Geometry check sheet. Reference: the model listing, model coordinates, mm. A direction names the side the tool comes from. Coordinates: 2 decimals unless noted, no trailing zeros. Loops run counter-clockwise (first coordinate to the right, second up) from the corner with the lowest first, then second, coordinate; pieces in that order, holes last.
from build123d import *

# Parameters (mm, degrees)
SKETCH_1_R          = 32.5
EXTRUDE_1_DEPTH     = 154.5
SKETCH_2_R          = 12.5
EXTRUDE_2_DEPTH     = 6
SKETCH_3_R          = 6
CUT_EXTRUDE_1_DEPTH = 80
SKETCH_4_R          = 8
EXTRUDE_3_DEPTH     = 5
SKETCH_5_R          = 8
EXTRUDE_4_DEPTH     = 2.5
SKETCH_8_R          = 4
SKETCH_7_R          = 6
SKETCH_9_R          = 2.5
CUT_EXTRUDE_2_DEPTH = 31
SKETCH_10_R         = 6
CUT_EXTRUDE_3_DEPTH = 17


with BuildPart() as part:
    # 草图1 → 凸台-拉伸1 (new body)
    with BuildSketch(Plane(origin=(0, 0, 0), x_dir=(1, 0, 0), z_dir=(0, 1, 0))):
        with Locations(Location((0, 0, 0), (0, 0, 270))):
            Circle(SKETCH_1_R)
    extrude(amount=EXTRUDE_1_DEPTH)

    # 草图2 → 凸台-拉伸2 (add)
    with BuildSketch(Plane.XZ):
        with Locations(Location((0, 0, 0), (0, 0, 270))):
            Circle(SKETCH_2_R)
    extrude(amount=EXTRUDE_2_DEPTH)

    # 草图3 → 切除-拉伸1 (cut)
    with BuildSketch(Plane.XZ.offset(6)):
        with Locations(Location((0, 0, 0), (0, 0, 270))):
            Circle(SKETCH_3_R)
    extrude(amount=-CUT_EXTRUDE_1_DEPTH, mode=Mode.SUBTRACT)

    # 草图4 → 凸台-拉伸3 (add, symmetric)
    with BuildSketch(Plane.XY):
        with BuildLine():
            Line((-11, 154.5), (11, 154.5))
            Line((11, 154.5), (11, 164.5))
            ThreePointArc((11, 164.5), (0, 175.5), (-11, 164.5))
            Line((-11, 164.5), (-11, 154.5))
        make_face()
        with Locations((0, 164.5)):
            Circle(SKETCH_4_R, mode=Mode.SUBTRACT)
    extrude(amount=EXTRUDE_3_DEPTH, both=True)

    # 草图5 → 凸台-拉伸4 (add, symmetric)
    with BuildSketch(Plane.XY):
        with Locations((0, 164.5)):
            Circle(SKETCH_5_R)
    extrude(amount=EXTRUDE_4_DEPTH, both=True)

    # 草图8 → 放样1 section 0
    with BuildSketch(Plane.XY.offset(4.5)):
        with Locations((0, 164.5)):
            Circle(SKETCH_8_R)
    # 草图7 → 放样1 section 1
    with BuildSketch(Plane.XY.offset(2.5)):
        with Locations((0, 164.5)):
            Circle(SKETCH_7_R)
    loft_1 = loft()

    # 镜向1: 放样1 across plane
    add(loft_1.mirror(Plane.XY))

    # 草图9 → 切除-拉伸2 (cut)
    with BuildSketch(Plane.XY.offset(4.5)):
        with Locations((0, 166.761335751)):
            Circle(SKETCH_9_R)
    extrude(amount=-CUT_EXTRUDE_2_DEPTH, mode=Mode.SUBTRACT)

    # 草图10 → 切除-拉伸3 (cut)
    with BuildSketch(Plane.XY.offset(4.5)):
        with Locations((0, 164.5)):
            Circle(SKETCH_10_R)
    extrude(amount=-CUT_EXTRUDE_3_DEPTH, mode=Mode.SUBTRACT)

    # 草图11 → 切除-旋转1 (revolve, cut)
    with BuildSketch(Plane.XY):
        with BuildLine():
            Line((0, 171), (0, 158))
            ThreePointArc((0, 158), (6.5, 164.5), (0, 171))
        make_face()
    revolve(axis=Axis((0, 171, 0), (0, -1, 0)), mode=Mode.SUBTRACT)


solid = part.part
(1) Gauge pin test, flat ends, axial feed: pin 1 Ø13 at (x, y) = (2.5, 162) entering from +Z; pin 2 Ø10.5 at (x, y) = (-0.5, 166.5) entering from -Z; pin 3 Ø8 at (y, z) = (63, -11) entering from -X. Record the tip position at first contact, or that the pin passes through.
Findings:
pin 1: stops at z = 5
pin 2: stops at z = -2.5
pin 3: stops at x = -31.74
(2) Draft check along X on faces 6 (the cylindrical face through (1.802, 33.44, -5.723)), 7 (the cylindrical face through (9.76, 76.17, 31)), 8 (the flat face through (0, 154.5, 7)). Enter one of: +X half, -X half, draft (parallel to the pull), parting line (faces both ways), or undercut.
Findings:
face 6: undercut
face 7: parting line
face 8: draft
(3) Scan lines: L1, parallel to Y at x = 0, z = 3.9; L2, parallel to X at y = 31, z = 0; L3, parallel to X at y = 164, z = -4. Record each from-to range of solid material in increasing order.
Findings:
L1: y = 74 to 156.5, 172.5 to 175.5
L2: x = -32.5 to -6, 6 to 32.5
L3: x = -11 to -7.98, 7.98 to 11
(4) Sectioned sample at D-D on x = 28. Record the cut outline in (y, z), and give its area (3 significant figures).
Findings:
outline: (0, -16.5) - (154.5, -16.5) - (154.5, 16.5) - (0, 16.5) - close
area: 5,100 mm2
(5) Sectioned sample at A-A on x = 0. Record the cut outline in (y, z), and give its area (3 significant figures).
Findings:
outline: (-6, -12.5) - (0, -12.5) - (0, -32.5) - (154.5, -32.5) - (154.5, -5) - (156.5, -5) - (156.5, -2.5) - (158.5, -2.5) arc R6.5 cw to (158.5, 2.5) - (156.5, 2.5) - (156.5, 5) - (154.5, 5) - (154.5, 32.5) - (0, 32.5) - (0, 12.5) - (-6, 12.5) - (-6, 6) - (74, 6) - (74, -6) - (-6, -6) - close; (170.5, -2.5) - (172.5, -2.5) - (172.5, -5) - (175.5, -5) - (175.5, 5) - (172.5, 5) - (172.5, 2.5) - (170.5, 2.5) arc R6.5 cw to start
area: 9,300 mm2
(6) Sectioned sample at B-B on z = 0. Record the cut outline in (x, y), and give its area (3 significant figures).
Findings:
outline: (-32.5, 0) - (-12.5, 0) - (-12.5, -6) - (-6, -6) - (-6, 74) - (6, 74) - (6, -6) - (12.5, -6) - (12.5, 0) - (32.5, 0) - (32.5, 154.5) - (11, 154.5) - (11, 164.5) arc R11 ccw to (-11, 164.5) - (-11, 154.5) - (-32.5, 154.5) - close; hole circle Ø13 at (0, 164.5)
area: 9,510 mm2
(7) Sectioned sample at C-C on y = 13. Record the cut outline in (x, z).
Findings:
outline: circle Ø65 at (0, 0); hole circle Ø12 at (0, 0)
(8) Access from +Z, -Z, +X, -X, +Y, -Y to the whole of each face (thin tool, end or side, straight path). Record for faces 1 (the flat face through (11, 159, 0)), 2 (the flat face through (-11, 160, 0)), 3 (the flat face through (0, 74, 0)), 4 (the flat face through (3, 170, 2.5)), 5 (the cylindrical face through (-1.73, 156.69, -3.77)).
Findings:
face 1: +Z, -Z, +X, +Y
face 2: +Z, -Z, -X, +Y
face 3: -Y
face 4: +Z
face 5: -Z
